from build123d import *

# Parameters (mm, degrees)
SKETCH_1_W          = 27
SKETCH_1_H          = 85
EXTRUDE_1_DEPTH     = 3
SKETCH_2_R          = 1.45
CUT_EXTRUDE_1_DEPTH = 90.235643103
CUT_EXTRUDE_2_DEPTH = 90.235643103
FILLET_1_R          = 10


with BuildPart() as part:
    # 草图1 → 凸台-拉伸1 (new body)
    with BuildSketch(Plane(origin=(0, 0, 0), x_dir=(1, 0, 0), z_dir=(0, 1, 0))):
        with Locations((13.5, 42.5)):
            Rectangle(SKETCH_1_W, SKETCH_1_H)
    extrude(amount=EXTRUDE_1_DEPTH)

    # 草图2 → 切除-拉伸1 (cut, through all)
    with BuildSketch(Plane(origin=(0, 3, 0), x_dir=(1, 0, 0), z_dir=(0, 1, 0))):
        with Locations(Location((6, 7.5, 0), (0, 0, 270))):
            Circle(SKETCH_2_R)
        with Locations(Location((21, 7.5, 0), (0, 0, 90))):
            Circle(SKETCH_2_R)
        with Locations(Location((21, 77.5, 0), (0, 0, 270))):
            Circle(SKETCH_2_R)
        with Locations(Location((6, 77.5, 0), (0, 0, 90))):
            Circle(SKETCH_2_R)
    extrude(amount=-CUT_EXTRUDE_1_DEPTH, mode=Mode.SUBTRACT)

    # 草图3 → 切除-拉伸2 (cut, through all)
    with BuildSketch(Plane(origin=(0, 3, 0), x_dir=(1, 0, 0), z_dir=(0, 1, 0))):
        with BuildLine():
            Line((10.5, 69.5), (10.5, 15.5))
            ThreePointArc((10.5, 15.5), (7.75, 12.75), (5, 15.5))
            Line((5, 15.5), (5, 69.5))
            ThreePointArc((5, 69.5), (7.75, 72.25), (10.5, 69.5))
        make_face()
        with BuildLine():
            Line((16.5, 69.5), (16.5, 15.5))
            ThreePointArc((16.5, 15.5), (19.25, 12.75), (22, 15.5))
            Line((22, 15.5), (22, 69.5))
            ThreePointArc((22, 69.5), (19.25, 72.25), (16.5, 69.5))
        make_face()
    extrude(amount=-CUT_EXTRUDE_2_DEPTH, mode=Mode.SUBTRACT)

    # 圆角1
    fillet_1_edges = [part.edges().sort_by_distance(p)[0] for p in [
        (0, 1.5, -85),
        (27, 1.5, -85),
        (27, 1.5, 0),
        (0, 1.5, 0),
    ]]
    fillet(fillet_1_edges, radius=FILLET_1_R)


solid = part.part
Design review of the part built by this model. Coordinates are the model's own, in mm. A direction names the side the tool comes from. Coordinates: 2 decimals unless noted, no trailing zeros. Order: outer loops, then holes, each group sorted by start corner. A loop starts at its lowest first (then second) coordinate and runs counter-clockwise, first axis right, second up. Notation, with made-up numbers: (26.5, -34.5) -> (71.5, -34.5) arc R8 cw to (71.5, -24.5) -> close; hole circle Ø7 at (-8.5, 29.5). An arc over 180 degrees is marked (long way). One line per item, written item: value.
1) Machinability: for faces 4 (the face through (19.31, 1.52, -72.25)), 5 (the face through (13, 3, -43)), which of the approach directions +Z, -Z, +X, -X, +Y, -Y give a long, thin tool a straight path to every point of the face, cutting with its end or side? Answer none if there is none.
Output values:
face 4: +Y, -Y
face 5: +Z, -Z, +X, -X, +Y
2) We need section B-B, the plane z = -63.5. Give the boundary of the cut face in (x, y), then the cut area to 3 significant figures.
Output values:
outline: (0, 0) -> (5, 0) -> (5, 3) -> (0, 3) -> close; (10.5, 0) -> (16.5, 0) -> (16.5, 3) -> (10.5, 3) -> close; (22, 0) -> (27, 0) -> (27, 3) -> (22, 3) -> close
area: 48.0 mm2
3) To check wall thickness, follow probe 1 along X at (y, z) = (0.3, -49.5); probe 2 along X at (y, z) = (2.05, -7); probe 3 along Z at (x, y) = (20.25, 1.5). State the ranges of each line that lie inside material, in increasing order. Write a range as [from, to].
Output values:
probe 1: x = [0, 5], [10.5, 16.5], [22, 27]
probe 2: x = [0.46, 4.64], [7.36, 19.64], [22.36, 26.54]
probe 3: z = [-84.46, -78.74], [-76.26, -72.06], [-12.94, -8.74], [-6.26, -0.54]
4) We need section C-C, the plane x = 21. Give the boundary of the cut face in (y, z).
Output values:
outline: (0, -84.17) -> (3, -84.17) -> (3, -78.95) -> (0, -78.95) -> close; (0, -76.05) -> (3, -76.05) -> (3, -71.62) -> (0, -71.62) -> close; (0, -13.38) -> (3, -13.38) -> (3, -8.95) -> (0, -8.95) -> close; (0, -6.05) -> (3, -6.05) -> (3, -0.83) -> (0, -0.83) -> close
5) We need section A-A, the plane y = 1.25. Give the boundary of the cut face in (x, z).
Output values:
outline: (0, -75) arc R10 ccw to (10, -85) -> (17, -85) arc R10 ccw to (27, -75) -> (27, -10) arc R10 ccw to (17, 0) -> (10, 0) arc R10 ccw to (0, -10) -> close; hole circle Ø2.9 at (6, -77.5); hole circle Ø2.9 at (6, -7.5); hole (5, -69.5) arc R2.75 ccw to (10.5, -69.5) -> (10.5, -15.5) arc R2.75 ccw to (5, -15.5) -> close; hole (16.5, -69.5) arc R2.75 ccw to (22, -69.5) -> (22, -15.5) arc R2.75 ccw to (16.5, -15.5) -> close; hole circle Ø2.9 at (21, -77.5); hole circle Ø2.9 at (21, -7.5)
6) Draft analysis for pull direction Z (two halves, no side actions). For faces 1 (the face through (10.5, 2, -43)), 2 (the face through (27, 1, -42)), 3 (the face through (13, 1, 0)), state which applies: +Z half, -Z half, draft (parallel to the pull), parting line (faces both ways), or undercut.
Output values:
face 1: undercut
face 2: draft
face 3: +Z half
7) We need section D-D, the plane z = -77.5. Give the boundary of the cut face in (x, y).
Output values:
outline: (0.32, 0) -> (4.55, 0) -> (4.55, 3) -> (0.32, 3) -> close; (7.45, 0) -> (19.55, 0) -> (19.55, 3) -> (7.45, 3) -> close; (22.45, 0) -> (26.68, 0) -> (26.68, 3) -> (22.45, 3) -> close
8) Clearance check with flat-ended pins moving along their axes: P1, Ø1.7, axis at x = 21, z = -77.5, coming from the +Y side; P2, Ø4.5, axis at x = 6, z = -7.5, coming from the +Y side. State where each tip first meets the part, or that it passes through.
Output values:
P1: passes through
P2: stops at y = 3
